```python
from build123d import *

# Parameters (mm, degrees)
SKETCH1_R                = 33
BOSS_EXTRUDE1_DEPTH      = 2
SKETCH2_R                = 3
BOSS_EXTRUDE2_DEPTH      = 2
FILLET1_R                = 5
CIRPATTERN1_COUNT        = 4
FILLET1_OF_CIRPATTERN1_R = 5
M3_CLEARANCE_HOLE1_D     = 3.4


with BuildPart() as part:
    # Sketch1 → Boss-Extrude1 (new body)
    with BuildSketch(Plane(origin=(0, 0, 0), x_dir=(1, 0, 0), z_dir=(0, 1, 0))):
        Circle(SKETCH1_R)
    extrude(amount=BOSS_EXTRUDE1_DEPTH)

    # Sketch2 → Boss-Extrude2 (add, through all)
    with BuildSketch(Plane(origin=(0, 2, 0), x_dir=(1, 0, 0), z_dir=(0, 1, 0))):
        with Locations((0, 34)):
            Circle(SKETCH2_R)
    boss_extrude2 = extrude(amount=-BOSS_EXTRUDE2_DEPTH)

    # Fillet1
    fillet1_edges = [part.edges().sort_by_distance(p)[0] for p in [
        (2.784037545, 1, -32.882352941),
        (-2.784037545, 1, -32.882352941),
    ]]
    fillet(fillet1_edges, radius=FILLET1_R)

    # CirPattern1: Boss-Extrude2 ×4 about axis
    cirpattern1_axis = Axis((0, 0, 0), (0, 1, 0))
    for i in range(1, CIRPATTERN1_COUNT):
        add(boss_extrude2.rotate(cirpattern1_axis, i * 360 / CIRPATTERN1_COUNT))

    # Fillet1 of CirPattern1
    fillet1_of_cirpattern1_edges = [part.edges().sort_by_distance(p)[0] for p in [
        (-32.882352941, 1, -2.784037545),
        (-32.882352941, 1, 2.784037545),
        (-2.784037545, 1, 32.882352941),
        (2.784037545, 1, 32.882352941),
        (32.882352941, 1, 2.784037545),
        (32.882352941, 1, -2.784037545),
    ]]
    fillet(fillet1_of_cirpattern1_edges, radius=FILLET1_OF_CIRPATTERN1_R)

    # M3 Clearance Hole1 (through all)
    with Locations(Plane(origin=(0, 2, 0), x_dir=(1, 0, 0), z_dir=(0, 1, 0))):
        with Locations((0, -34), (34, 0), (0, 34), (-34, 0)):
            Hole(M3_CLEARANCE_HOLE1_D / 2)


solid = part.part
```
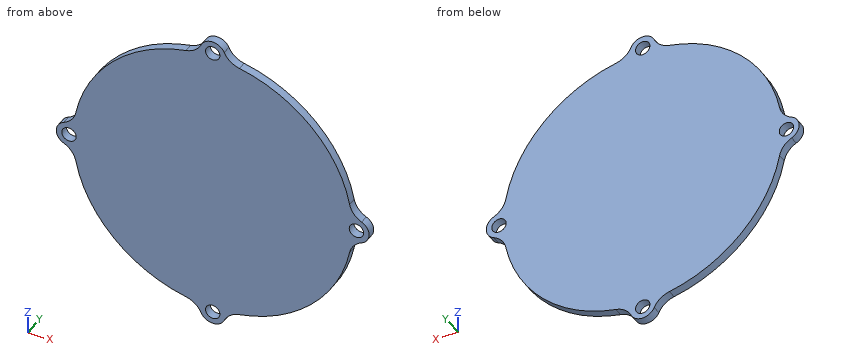
Part model, mm, in its own coordinate system. Round coordinates to 2 decimals unless told otherwise and drop trailing zeros. Order: outer loops, then holes, each group sorted by start corner. A loop starts at its lowest first (then second) coordinate and runs counter-clockwise, first axis right, second up. Notation, with made-up numbers: M 59,65.25 L 88,65.25 A13 cw 88,73.25 Z; hole C 67.5,72.5 d5. An arc over 180 degrees is marked long. Put each result on its own line as item: value. Start each with the question number.
1. Slice it at B-B on z = 0. List the corners of the cut face in (x, y).
2. Slice it at D-D on z = -9.5. List the corners of the cut face in (x, y).
3. Drop a flat-ended pin along its axis: pin 1 (2 mm diameter, centred on x = 34, z = 0, fed in from +Y). Give the stop position or say it passes through.
4. Drill centre lines: probe 1 along Z at (x, y) = (0, 0.45); probe 2 along X at (y, z) = (0.85, 1); probe 3 along Z at (x, y) = (34, 0.75). Where is each one in solid material? Low to high. Write a range as [from, to].
5. Slice it at C-C on y = 0.8. State how many separate pieces and enclosed holes the cut face has, then the cut area to 3 significant figures.
6. Slice it at A-A on x = 0. List the corners of the cut face in (y, z).
Findings:
1. outline: M -37,0 L -35.7,0 L -35.7,2 L -37,2 Z; M -32.3,0 L 32.3,0 L 32.3,2 L -32.3,2 Z; M 35.7,0 L 37,0 L 37,2 L 35.7,2 Z
2. outline: M -31.6,0 L 31.6,0 L 31.6,2 L -31.6,2 Z
3. pin 1: through
4. probe 1: [-37, -35.7], [-32.3, 32.3], [35.7, 37]
4. probe 2: [-36.83, -35.37], [-32.63, 32.63], [35.37, 36.83]
4. probe 3: [-3.53, -1.7], [1.7, 3.53]
5. separate pieces: 1
5. enclosed holes: 4
5. area: 3,480 mm2
6. outline: M 0,-37 L 2,-37 L 2,-35.7 L 0,-35.7 Z; M 0,-32.3 L 2,-32.3 L 2,32.3 L 0,32.3 Z; M 0,35.7 L 2,35.7 L 2,37 L 0,37 Z
